from build123d import *

# Parameters (mm, degrees)
F0_W     = 82.55
F0_H     = 38.1
F1_DEPTH = 82.55
F3_T     = -2.54
F5_D     = 7.9375
F5_DEPTH = 12.7
F6_W     = 15.181465
F6_H     = 8.003246
F7_DEPTH = 2.54


with BuildPart() as f1:
    # F0 (on Front) → F1 (new body)
    with BuildSketch(Plane.XZ):
        with Locations((41.275, 19.05)):
            Rectangle(F0_W, F0_H)
    extrude(amount=F1_DEPTH)

    # F3
    f3_openings = [f1.faces().sort_by_distance(p)[0] for p in [
        (41.275, -41.275, 38.1),
    ]]
    offset(amount=F3_T, openings=f3_openings)

    # F5
    with Locations(Plane.XZ.offset(82.55)):
        with Locations((40.470496, 20.613467)):
            Hole(F5_D / 2, depth=F5_DEPTH)

    # F6 (on face) → F7 (cut, through all)
    with BuildSketch(Plane.XZ.offset(82.55)):
        with Locations((15.511802, 19.324051)):
            Rectangle(F6_W, F6_H)
    extrude(amount=-F7_DEPTH, mode=Mode.SUBTRACT)


solid = f1.part
Part model, mm, in its own coordinate system. A direction names the side the tool comes from. Give positions to 0.01 mm unless a question says otherwise; leave off trailing zeros. Write each loop counter-clockwise with the first axis right and the second up, starting at its lowest first coordinate (ties: lowest second). Pieces come first, ordered by that corner, then holes.
1) Cut at C-C on z = 33.5. Write the cut outline in (x, y).
Resolved:
outline: (0, -82.55) - (82.55, -82.55) - (82.55, 0) - (0, 0) - close; hole (2.54, -80.01) - (80.01, -80.01) - (80.01, -2.54) - (2.54, -2.54) - close
2) Two-plate mould, pull along Z, no slides. Class faces 1 (the face through (41, -2.54, 21)), 2 (the face through (38, -81, 38.1)), 3 (the face through (23.103, -81, 19)), 4 (the face through (41.33, -81.26, 16.74)): released by +Z, released by -Z, zero draft, split by the parting line, or undercut.
Resolved:
face 1: zero draft
face 2: released by +Z
face 3: undercut
face 4: undercut
3) Cut at D-D on x = 47.5. Write the cut outline in (y, z), then the cut area to 3 significant figures.
Resolved:
outline: (-82.55, 0) - (0, 0) - (0, 38.1) - (-2.54, 38.1) - (-2.54, 2.54) - (-80.01, 2.54) - (-80.01, 38.1) - (-82.55, 38.1) - close
area: 390 mm2
4) Cut at B-B on y = -57. Write the cut outline in (x, z).
Resolved:
outline: (0, 0) - (82.55, 0) - (82.55, 38.1) - (80.01, 38.1) - (80.01, 2.54) - (2.54, 2.54) - (2.54, 38.1) - (0, 38.1) - close
5) Cut at A-A on x = 16. Write the cut outline in (y, z).
Resolved:
outline: (-82.55, 0) - (0, 0) - (0, 38.1) - (-2.54, 38.1) - (-2.54, 2.54) - (-80.01, 2.54) - (-80.01, 15.32) - (-82.55, 15.32) - close; (-82.55, 23.33) - (-80.01, 23.33) - (-80.01, 38.1) - (-82.55, 38.1) - close
6) Pin check, flat tips, straight feed: pin 1 (9 mm diameter, centred on x = 40.47, z = 20.61, fed in from +Y); pin 2 (8 mm diameter, centred on x = 23.5, y = -31.5, fed in from +Z). Stop position of each tip, or through.
Resolved:
pin 1: stops at y = 0
pin 2: stops at z = 2.54
7) Which spindle directions (+Z, -Z, +X, -X, +Y, -Y) get a long thin tool onto all of the face, cutting with end or side? Do faces 5 (the face through (82.55, -41, 19)), 6 (the face through (41, -41, 2.54)), 7 (the face through (15, -81, 23.326)). Say none if no direction does.
Resolved:
face 5: +Z, -Z, +X, +Y, -Y
face 6: +Z
face 7: -Y
8) Probe L1, parallel to Y at x = 64.5, z = 3; L2, parallel to X at y = -73, z = 20; L3, parallel to Z at x = 10, y = -16. List the from-to ranges inside material, lowest first.
Resolved:
L1: y = -82.55 to -80.01, -2.54 to 0
L2: x = 0 to 2.54, 80.01 to 82.55
L3: z = 0 to 2.54
